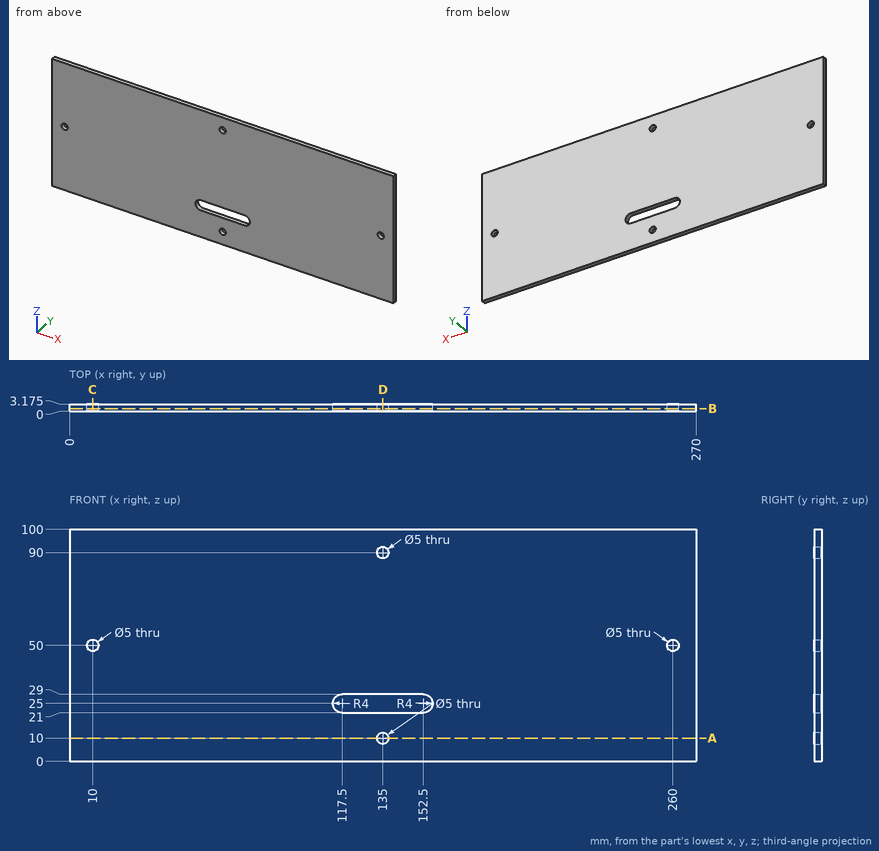
Could you check a few things on this drawing? It's one solid part, dimensions in mm from its lowest x, y, z. Round coordinates to 2 decimals unless told otherwise and drop trailing zeros. Order: outer loops, then holes, each group sorted by start corner. A loop starts at its lowest first (then second) coordinate and runs counter-clockwise, first axis right, second up. Notation, with made-up numbers: M 21.5,14.5 L 30.5,14.5 A18 ccw 30.5,47.5 Z; hole C 59.25,17 d7. An arc over 180 degrees is marked long. One line per question, with ' | ' between items. Start each with the question number.
(1) Please list where these lines run through material, in increasing order: line 1 along X through (y, z) = (2.4, 50); line 2 along Z through (x, y) = (135, 1.75); line 3 along X through (y, z) = (2.5, 10).
(2) Suppose I cut it at D-D on x = 135. List the corners of the cut face in (y, z) for me (3 decimals), then the cut area to 3 significant figures.
(3) For P1, Ø4, axis at x = 10, z = 50, coming from the -Y side, with a flat end and sliding along its axis, tell me the tip position at first contact or that it passes through.
(4) Suppose I cut it at B-B on y = 1.2. List the corners of the cut face in (x, z) for me.
(5) Suppose I cut it at A-A on z = 10. List the corners of the cut face in (x, y) for me (3 decimals), then the cut area to 3 significant figures.
(6) Suppose I cut it at C-C on x = 10. List the corners of the cut face in (y, z) for me (3 decimals), then the cut area to 3 significant figures.
Geometry results:
1) line 1: 0 to 7.5, 12.5 to 257.5, 262.5 to 270 | line 2: 0 to 7.5, 12.5 to 21, 29 to 87.5, 92.5 to 100 | line 3: 0 to 132.5, 137.5 to 270
2) outline: M 0,0 L 3.175,0 L 3.175,7.5 L 0,7.5 Z; M 0,12.5 L 3.175,12.5 L 3.175,21 L 0,21 Z; M 0,29 L 3.175,29 L 3.175,87.5 L 0,87.5 Z; M 0,92.5 L 3.175,92.5 L 3.175,100 L 0,100 Z | area: 260 mm²
3) P1: through
4) outline: M 0,0 L 270,0 L 270,100 L 0,100 Z; hole C 10,50 d5; hole M 117.5,21 L 152.5,21 A4 ccw 152.5,29 L 117.5,29 A4 ccw Z; hole C 135,10 d5; hole C 135,90 d5; hole C 260,50 d5
5) outline: M 0,0 L 132.5,0 L 132.5,3.175 L 0,3.175 Z; M 137.5,0 L 270,0 L 270,3.175 L 137.5,3.175 Z | area: 841 mm²
6) outline: M 0,0 L 3.175,0 L 3.175,47.5 L 0,47.5 Z; M 0,52.5 L 3.175,52.5 L 3.175,100 L 0,100 Z | area: 302 mm²
